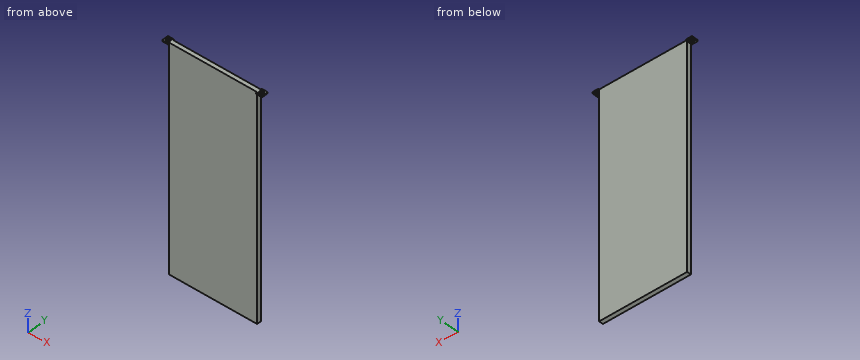
from build123d import *

# Parameters (mm, degrees)
SKETCH1_W           = 210.28
SKETCH1_H           = 10
BOSS_EXTRUDE1_DEPTH = 531
SKETCH2_W           = 3
SKETCH2_H           = 15
BOSS_EXTRUDE2_DEPTH = 14
SKETCH4_W           = 3
SKETCH4_H           = 15
BOSS_EXTRUDE3_DEPTH = 14
SKETCH3_R           = 4.7
CUT_EXTRUDE1_DEPTH  = 13


with BuildPart() as part:
    # Sketch1 → Boss-Extrude1 (new body)
    with BuildSketch(Plane.XY):
        with Locations((105.14, 5)):
            Rectangle(SKETCH1_W, SKETCH1_H)
    extrude(amount=BOSS_EXTRUDE1_DEPTH)

    # Sketch2 → Boss-Extrude2 (add)
    with BuildSketch(Plane.ZY):
        with Locations((529.5, 5)):
            Rectangle(SKETCH2_W, SKETCH2_H)
    extrude(amount=BOSS_EXTRUDE2_DEPTH)

    # Sketch4 → Boss-Extrude3 (add)
    with BuildSketch(Plane(origin=(210.28, 0, 0), x_dir=(0, 0, -1), z_dir=(1, 0, 0))):
        with Locations((-529.5, 5)):
            Rectangle(SKETCH4_W, SKETCH4_H)
    extrude(amount=BOSS_EXTRUDE3_DEPTH)

    # Sketch3 → Cut-Extrude1 (cut)
    with BuildSketch(Plane(origin=(0, 0, 528), x_dir=(-1, 0, 0), z_dir=(0, 0, -1))):
        with Locations((6.5, 5)):
            Circle(SKETCH3_R)
        with Locations((-216.78, 5)):
            Circle(SKETCH3_R)
    extrude(amount=-CUT_EXTRUDE1_DEPTH, mode=Mode.SUBTRACT)


solid = part.part
The listing builds one solid part. Answer for the finished solid, in the listing's coordinates (mm). Give positions to 0.01 mm unless a question says otherwise; leave off trailing zeros. Order: outer loops, then holes, each group sorted by start corner. A loop starts at its lowest first (then second) coordinate and runs counter-clockwise, first axis right, second up. Notation, with made-up numbers: (-18.75, -10) - (-14.75, -10) arc R20 ccw to (-14.75, 11) - close; hole circle Ø4 at (59, -34.5). An arc over 180 degrees is marked (long way). Use one line per item in the form item = value.
1) Find section B-B on x = -6.5. Determine the outline of the cut face in (y, z).
Verdict:
outline = (-2.5, 528) - (0.3, 528) - (0.3, 531) - (-2.5, 531) - close; (9.7, 528) - (12.5, 528) - (12.5, 531) - (9.7, 531) - close
2) Consider probe 1 along Y at (x, z) = (216, 529); probe 2 along Y at (x, z) = (216.78, 529.3); probe 3 along Y at (x, z) = (207.5, 49.5). Determine where each line is inside the solid, lowest interval first. Write a range as [from, to].
Verdict:
probe_1 = [-2.5, 0.37], [9.63, 12.5]
probe_2 = [-2.5, 0.3], [9.7, 12.5]
probe_3 = [0, 10]
3) Find section D-D on z = 444. Determine the outline of the cut face in (x, y), and give its area (3 significant figures).
Verdict:
outline = (0, 0) - (210.28, 0) - (210.28, 10) - (0, 10) - close
area = 2,100 mm^2
4) Find section A-A on y = 5. Determine the outline of the cut face in (x, z).
Verdict:
outline = (-14, 528) - (-11.2, 528) - (-11.2, 531) - (-14, 531) - close; (-1.8, 528) - (0, 528) - (0, 0) - (210.28, 0) - (210.28, 528) - (212.08, 528) - (212.08, 531) - (-1.8, 531) - close; (221.48, 528) - (224.28, 528) - (224.28, 531) - (221.48, 531) - close
5) Each of these flat-tipped pins is pushed along its axis until it touches: pin 1 (1 mm diameter, centred on x = 103, z = 178.5, fed in from +Y); pin 2 (2 mm diameter, centred on y = 9, z = 455, fed in from +X); pin 3 (2 mm diameter, centred on x = 187, z = 419, fed in from -Y); pin 4 (3 mm diameter, centred on x = 91, y = 11, fed in from -Z). Where does it stop, or does it pass through?
Verdict:
pin_1 = 10
pin_2 = 210.28
pin_3 = 0
pin_4 = 0
6) Find section C-C on x = 67.5. Determine the outline of the cut face in (y, z), and give its area (3 significant figures).
Verdict:
outline = (0, 0) - (10, 0) - (10, 531) - (0, 531) - close
area = 5,310 mm^2
